```python
from build123d import *

# Parameters (mm, degrees)
SKETCH_1_W               = 28.4
SKETCH_1_H               = 30
EXTRUDE_1_DEPTH          = 3
SKETCH_2_R               = 6.55
CUT_EXTRUDE_1_DEPTH      = 3
SKETCH_3_R               = 1.525
CUT_EXTRUDE_2_DEPTH      = 3
PATTERN_CIRCULAR_1_COUNT = 6
SKETCH_4_W               = 8
SKETCH_4_H               = 3
EXTRUDE_2_DEPTH          = 3
SKETCH_5_R               = 1.05
CUT_EXTRUDE_3_DEPTH      = 3
SKETCH_6_W               = 18
SKETCH_6_H               = 6
EXTRUDE_3_DEPTH          = 3
SKETCH_7_R               = 1.025
CUT_EXTRUDE_4_DEPTH      = 3


with BuildPart() as part:
    # 草图1 → 凸台-拉伸1 (new body)
    with BuildSketch(Plane.XY):
        Rectangle(SKETCH_1_W, SKETCH_1_H)
    extrude(amount=EXTRUDE_1_DEPTH)

    # 草图2 → 切除-拉伸1 (cut)
    with BuildSketch(Plane.XY.offset(3)):
        with Locations((0, 1.5)):
            Circle(SKETCH_2_R)
    extrude(amount=-CUT_EXTRUDE_1_DEPTH, mode=Mode.SUBTRACT)

    # 草图3 → 切除-拉伸2 (cut)
    with BuildSketch(Plane.XY.offset(3)):
        with Locations((-9.5, 1.5)):
            Circle(SKETCH_3_R)
    cut_extrude_2 = extrude(amount=-CUT_EXTRUDE_2_DEPTH, mode=Mode.SUBTRACT)

    # 阵列(圆周)1: 切除-拉伸2 ×6 about axis
    pattern_circular_1_axis = Axis((0, 1.5, 0), (0, 0, 1))
    for i in range(1, PATTERN_CIRCULAR_1_COUNT):
        add(cut_extrude_2.rotate(pattern_circular_1_axis, i * 360 / PATTERN_CIRCULAR_1_COUNT), mode=Mode.SUBTRACT)

    # 草图4 → 凸台-拉伸2 (add)
    with BuildSketch(Plane(origin=(0, 0, 0), x_dir=(-1, 0, 0), z_dir=(0, 0, -1))):
        with Locations((-10.2, 16.5)):
            Rectangle(SKETCH_4_W, SKETCH_4_H)
        with Locations((10.2, 16.5)):
            Rectangle(SKETCH_4_W, SKETCH_4_H)
    extrude(amount=-EXTRUDE_2_DEPTH)

    # 草图5 → 切除-拉伸3 (cut)
    with BuildSketch(Plane.XY.offset(3)):
        with Locations((-5.15, 15)):
            Circle(SKETCH_5_R)
        with Locations((5.15, 15)):
            Circle(SKETCH_5_R)
    extrude(amount=-CUT_EXTRUDE_3_DEPTH, mode=Mode.SUBTRACT)

    # 草图6 → 凸台-拉伸3 (add)
    with BuildSketch(Plane(origin=(0, 0, 0), x_dir=(-1, 0, 0), z_dir=(0, 0, -1))):
        with Locations((0, -15)):
            Rectangle(SKETCH_6_W, SKETCH_6_H)
    extrude(amount=-EXTRUDE_3_DEPTH)

    # 草图7 → 切除-拉伸4 (cut)
    with BuildSketch(Plane(origin=(0, 0, 0), x_dir=(-1, 0, 0), z_dir=(0, 0, -1))):
        with Locations((10.025, -15)):
            Circle(SKETCH_7_R)
        with Locations((-10.025, -15)):
            Circle(SKETCH_7_R)
    extrude(amount=-CUT_EXTRUDE_4_DEPTH, mode=Mode.SUBTRACT)


solid = part.part
```
Design review of the part built by this model. Coordinates are the model's own, in mm. A direction names the side the tool comes from. Round coordinates to 2 decimals unless told otherwise and drop trailing zeros. Write each loop counter-clockwise with the first axis right and the second up, starting at its lowest first coordinate (ties: lowest second). Pieces come first, ordered by that corner, then holes.
Item 1: For probe 1 along Y at (x, z) = (0, 1.3); probe 2 along X at (y, z) = (16, 2.4); probe 3 along X at (y, z) = (9, 1.75), list the stretches that pass through material, from the lowest coordinate up.
Item 2: Clearance check with flat-ended pins moving along their axes: pin 1 Ø17 at (x, y) = (0, 1.5) entering from -Z; pin 2 Ø0.9 at (x, z) = (-12, 2) entering from -Y; pin 3 Ø0.9 at (x, z) = (-0.5, 1) entering from +Y; pin 4 Ø1.5 at (x, z) = (-10, 1) entering from -Y. State where each tip first meets the part, or that it passes through.
Item 3: We need section B-B on x = 0. Write out the cut boundary in (y, z).
Item 4: For faces 5 (the flat face through (0, 15, 1)), 6 (the flat face through (9, -17, 1)), 7 (the cylindrical face through (4.551, -5.215, 1.521)), 8 (the flat face through (-13, -15, 1)), list the 3-axis set-ups (+Z, -Z, +X, -X, +Y, -Y) from which the entire face can be reached by the end or side of a thin tool; tool diameter is ignored.
Item 5: We need section D-D on x = 5.15. Write out the cut boundary in (y, z), and give its area (3 significant figures).
Item 6: We need section A-A on y = 1.5. Write out the cut boundary in (x, z) (3 decimals).
Item 7: The part is to be moulded in two halves that separate along Y. For faces 1 (the cylindrical face through (-10.048, -13.975, 1.479)), 2 (the flat face through (6.2, 16, 1)), 3 (the flat face through (-10, 18, 1)), 4 (the cylindrical face through (8.045, 1.042, 1.521)), say which applies: +Y half, -Y half, draft (parallel to the pull), parting line (faces both ways), or undercut.
Item 8: We need section C-C on y = -7. Write out the cut boundary in (x, z), and give its area (3 significant figures).
Returned:
1. probe 1: y = -18 to -5.05, 8.05 to 15
1. probe 2: x = -14.2 to -6.2, 6.2 to 14.2
1. probe 3: x = -14.2 to -6.09, -3.41 to 3.41, 6.09 to 14.2
2. pin 1: stops at z = 0
2. pin 2: stops at y = -15
2. pin 3: stops at y = 15
2. pin 4: stops at y = -14.33
3. outline: (-18, 0) - (-5.05, 0) - (-5.05, 3) - (-18, 3) - close; (8.05, 0) - (15, 0) - (15, 3) - (8.05, 3) - close
4. face 5: +Z, -Z, +Y
4. face 6: +Z, -Z, +X, -Y
4. face 7: +Z, -Z
4. face 8: +Z, -Z, -X, -Y
5. outline: (-18, 0) - (-8.2, 0) - (-8.2, 3) - (-18, 3) - close; (-5.26, 0) - (-2.55, 0) - (-2.55, 3) - (-5.26, 3) - close; (5.55, 0) - (8.26, 0) - (8.26, 3) - (5.55, 3) - close; (11.2, 0) - (13.95, 0) - (13.95, 3) - (11.2, 3) - close
5. area: 53.9 mm2
6. outline: (-14.2, 0) - (-11.025, 0) - (-11.025, 3) - (-14.2, 3) - close; (-7.975, 0) - (-6.55, 0) - (-6.55, 3) - (-7.975, 3) - close; (6.55, 0) - (7.975, 0) - (7.975, 3) - (6.55, 3) - close; (11.025, 0) - (14.2, 0) - (14.2, 3) - (11.025, 3) - close
7. face 1: -Y half
7. face 2: draft
7. face 3: +Y half
7. face 4: undercut
8. outline: (-14.2, 0) - (-6.25, 0) - (-6.25, 3) - (-14.2, 3) - close; (-3.25, 0) - (3.25, 0) - (3.25, 3) - (-3.25, 3) - close; (6.25, 0) - (14.2, 0) - (14.2, 3) - (6.25, 3) - close
8. area: 67.2 mm2
